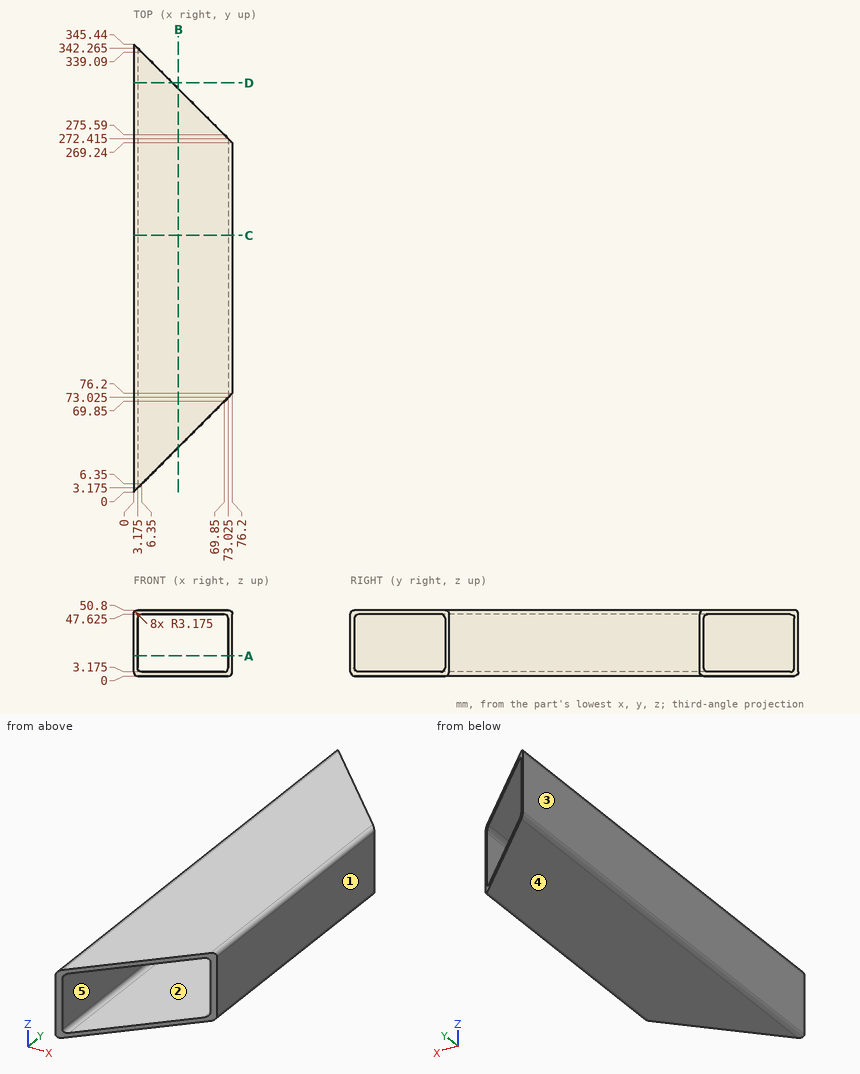
For this review, use the dimensioned drawing (mm, ordinates from the lowest corner) and the shaded views. A direction names the side the tool comes from. Give positions to 0.01 mm unless a question says otherwise; leave off trailing zeros. Order: outer loops, then holes, each group sorted by start corner. A loop starts at its lowest first (then second) coordinate and runs counter-clockwise, first axis right, second up. Notation, with made-up numbers: M 35,-11.5 L 94,-11.5 A11 ccw 94,9.5 Z; hole C 80.25,6 d7. An arc over 180 degrees is marked long. Use one line per item in the form item = value. Start each with the question number.
Item 1: For the marked faces 1 and 2, list the 3-axis set-ups (+Z, -Z, +X, -X, +Y, -Y) from which the entire face can be reached by the end or side of a thin tool; tool diameter is ignored.
Item 2: To check wall thickness, follow line 1 along Z through (x, y) = (14.5, 184) (3 decimals); line 2 along X through (y, z) = (125.5, 32.5) (3 decimals); line 3 along X through (y, z) = (314, 25) (3 decimals). State the ranges of each line that lie inside material, in increasing order. Write a range as from..to.
Item 3: We need section C-C on y = 198. Give the boundary of the cut face in (x, z) (3 decimals).
Item 4: Insertion check: pin 1 Ø2 at (y, z) = (90.5, 24) entering from -X. The pin has a flat end and moves straight along its axis. Give the tip position at first contact, or say it passes through.
Item 5: The part is to be moulded in two halves that separate along Z. For the marked faces 3, 4 and 5, say which applies: pulls with the +Z half, pulls with the -Z half, needs draft (parallel to the pull), parting line crosses it, or undercut.
Item 6: We need section A-A on z = 15.5. Give the boundary of the cut face in (x, y) (3 decimals), plus the area to 3 significant figures.
Item 7: We need section D-D on y = 315.5. Give the boundary of the cut face in (x, z) (3 decimals), plus the area to 3 significant figures.
Item 8: We need section B-B on x = 34.5. Give the boundary of the cut face in (y, z) (3 decimals), plus the area to 3 significant figures.
Completed:
q1.face_1 = +Z, -Z, +X, +Y, -Y
q1.face_2 = +Y, -Y
q2.line_1 = 0..3.175, 47.625..50.8
q2.line_2 = 0..3.175, 73.025..76.2
q2.line_3 = 0..3.175
q3.outline = M 0,3.175 A3.175 ccw 3.175,0 L 73.025,0 A3.175 ccw 76.2,3.175 L 76.2,47.625 A3.175 ccw 73.025,50.8 L 3.175,50.8 A3.175 ccw 0,47.625 Z; hole M 3.175,6.35 A3.175 ccw 6.35,3.175 L 69.85,3.175 A3.175 ccw 73.025,6.35 L 73.025,44.45 A3.175 ccw 69.85,47.625 L 6.35,47.625 A3.175 ccw 3.175,44.45 Z
q4.pin_1 = 0
q5.face_3 = needs draft
q5.face_4 = pulls with the -Z half
q5.face_5 = undercut
q6.outline = M 0,0 L 3.175,3.175 L 3.175,342.265 L 0,345.44 Z; M 73.025,73.025 L 76.2,76.2 L 76.2,269.24 L 73.025,272.415 Z
q6.area = 1,710 mm²
q7.outline = M 0,3.175 A3.175 ccw 3.175,0 L 29.94,0 L 29.94,3.175 L 6.35,3.175 A3.175 cw 3.175,6.35 L 3.175,44.45 A3.175 cw 6.35,47.625 L 29.94,47.625 L 29.94,50.8 L 3.175,50.8 A3.175 ccw 0,47.625 Z
q7.area = 331 mm²
q8.outline = M 34.5,0 L 310.94,0 L 310.94,3.175 L 34.5,3.175 Z; M 34.5,47.625 L 310.94,47.625 L 310.94,50.8 L 34.5,50.8 Z
q8.area = 1,760 mm²
